Autodesk Inventor part; units mm, degrees
ref_plane "Work Plane1" through (46.6583, 0, 0) normal (0, 0, -1) x (1, 0, 0)
ref_plane "YZ Plane" through (0, 0, 0) normal (1, 0, 0) x (0, 1, 0)
ref_plane "XZ Plane" through (0, 0, 0) normal (0, 1, 0) x (-1, 0, 0)
sketch "Sketch1" plane through (0, 0, 0) normal (0, 0, 1) x (1, 0, 0)
  line L0 (0, 0) -> (10, 0)
  line L1 (0, 0) -> (0, 8)
  line L2 (10, 6.25) -> (10, 0)
  line L3 (0, 8) -> (9.7606, 17.7458)
  line L4 (10, 6.25) -> (15.5202, 7.6958)
  arc A0 (15.5202, 7.6958) -> (9.7606, 17.7458) centre (14, 13.5) ccw
  line L5 (10, 6.25) -> (0, 8)
  line L6 (10, 6.25) -> (0, 3.6309)
  dimension "d0" = 12.5
  dimension "d1" = 14
  dimension "d2" = 13.5
  dimension "d3" = 6
  dimension "d4" = 10
  dimension "d5" = 16
revolve "Body" add sketch "Sketch1" angle 360 about axis through (0, 0, 0) along (1, 0, 0) contours L1 L6 L2 L0 | L1 L5 L6
extrude "Wing1" add sketch "Sketch1" along normal mid plane 2.8 contours L1 L5 L6 | L5 L3 A0 L4
fillet "Fillet1" [suppressed]
mirror "Wing2" about plane through (0, 0, 0) normal (0, 1, 0) of "Wing1"
sketch "Sketch2" plane through (0, 0, 0) normal (1, 0, 0) x (0, 1, 0)
  line L0 (0, -14) -> (0, 14)
  line L1 (-14, 0) -> (14, 0)
  point P0 (0, 0)
hole "Thread" at (0, 0, 0) direction (1, 0, 0) diameter 6.647 end through all
chamfer "Chamfer1" distance 0.6766 angle 30 1 edges at (0, 0, -3.3235) measured on face at (0, -6.3508, -0.1335)
ref_plane "Work Plane1" through (46.6583, 0, 0) normal (0, 0, -1) x (1, 0, 0)
equation "\"d0\" = KOD2"
equation "\"d1\" = KOH1 - RR"
equation "\"d2\" = 0.5 * E0 - RR"
equation "\"d3\" = RR"
equation "\"d4\" = KOH"
equation "\"d5\" = KOD"
equation "\"d6\" = SW"
equation "\"d8\" = 0.333333 * SW"
equation "\"d9\" = -0.5 * GD1 + 0.5 * NND"
equation "\"d109\" = -0.5 * GD1 + 0.5 * NND"
equation "\"NND\" = 8"
equation "\"KOH\" = 10"
equation "\"KOH1\" = 20"
equation "\"SW\" = 2.8"
equation "\"KOD\" = 16"
equation "\"KOD2\" = 12.5"
equation "\"RR\" = 6"
equation "\"E0\" = 39"
equation "\"GUL\" = 0.541266 * PTC"
equation "\"BOR\" = 0"
equation "\"PTC\" = 1.25"
equation "\"THREADDIA\" = 8"
equation "\"TOA\" = 30deg"
equation "\"RR2\" = 3"
equation "\"SW1\" = 4.4"
equation "\"GAL\" = 0.541266 * PTC"
properties part number "DIN 315 - M8" material "Steel, Mild"
Source: CAD feature listing. Evaluate the final solid. Frame: model axes, mm. A direction names the side the tool comes from. Round coordinates to 2 decimals unless told otherwise and drop trailing zeros. Write each loop counter-clockwise with the first axis right and the second up, starting at its lowest first coordinate (ties: lowest second). Pieces come first, ordered by that corner, then holes. Notation, with made-up numbers: M -34.75,13 L -21.75,13 A29 cw -21.75,34 Z; hole C 3,4.5 d4. An arc over 180 degrees is marked long. Answer as a JSON object with one key per item and string values. Group by question number.
(1) Section query C-C on y = 16.5. Output: boundary loops of the cut face in (x, z).
(2) Section query B-B on x = 14. Output: boundary loops of the cut face in (y, z).
(3) First-contact query: pin 1 (6 mm diameter, centred on x = 15, y = 9, fed in from +Z); pin 2 (2 mm diameter, centred on x = 2.5, z = -2.5, fed in from -Y); pin 3 (6 mm diameter, centred on y = 2.5, z = -0.5, fed in from +X). Flat tips, straight axial feed; report the tip coordinate or a pass-through.
(4) Ray query, line 1 (Y direction, x = 3.25, z = 0); line 2 (Z direction, x = 5.25, y = 0); line 3 (Y direction, x = 4, z = 0). Return the intervals inside material, ascending. Write a range as [from, to].
(5) Mould query, pull axis Z, two halves, no side actions, for faces 1 (the flat face through (12, -13, -1.4)), 2 (the flat face through (4.95, -12.94, -0.02)), 3 (the cylindrical face through (5.26, 1.27, 3.07)). Classes: +Z half, -Z half, draft (parallel to the pull), parting line (faces both ways), or undercut.
(6) Section query D-D on y = -13.5. Output: boundary loops of the cut face in (x, z).
(7) Reachability of faces 4 (the flat face through (10, 3, -3)), 5 (the cylindrical face through (19.28, -16.35, -0.02)) from +Z, -Z, +X, -X, +Y, -Y: full face, straight path, thin tool, end or side. Return the list, or none.
(8) Section query A-A on y = 0. Output: boundary loops of the cut face in (x, z).
Computed values:
{
 "1": {"outline": "M 8.51,-1.4 L 19.2,-1.4 L 19.2,1.4 L 8.51,1.4 Z"},
 "2": {"outline": "M -19.5,-1.4 L -7.3,-1.4 L -7.3,1.4 L -19.5,1.4 Z; M 7.3,-1.4 L 19.5,-1.4 L 19.5,1.4 L 7.3,1.4 Z"},
 "3": {"pin 1": "z = 1.4", "pin 2": "y = -7.48", "pin 3": "x = 10"},
 "4": {"line 1": "[-11.25, -3.32], [3.32, 11.25]", "line 2": "[-7.08, -3.32], [3.32, 7.08]", "line 3": "[-11.99, -3.32], [3.32, 11.99]"},
 "5": {"face 1": "-Z half", "face 2": "draft", "face 3": "undercut"},
 "6": {"outline": "M 5.51,-1.4 L 20,-1.4 L 20,1.4 L 5.51,1.4 Z"},
 "7": {"face 4": "+Z, -Z, +X", "face 5": "+Z, -Z"},
 "8": {"outline": "M 0,-8 L 10,-6.25 L 10,-3.32 L 0.39,-3.32 L 0,-4 Z; M 0,4 L 0.39,3.32 L 10,3.32 L 10,6.25 L 0,8 Z"}
}
